Input: dimensioned drawing with shaded views. Units: mm. Origin: part minimum x, y, z. Give positions to 0.01 mm unless a question says otherwise; leave off trailing zeros. Write each loop counter-clockwise with the first axis right and the second up, starting at its lowest first coordinate (ties: lowest second). Pieces come first, ordered by that corner, then holes.
Q1. Mould query, pull axis X, two halves, no side actions, for the marked faces 1, 2 and 3. Classes: +X half, -X half, draft (parallel to the pull), parting line (faces both ways), or undercut.
Q2. Section C-C (z = 24.5). Return the cut outline in (x, y), plus the area to 3 significant figures.
Q3. Line query: line 1 (X direction, y = 50, z = 18.5); line 2 (Z direction, x = 92, y = 27). Output: solid intervals per line, ascending.
Q4. Section A-A (y = 50). Return the cut outline in (x, z).
Q5. Pin query (flat end, axial travel): pin 1 Ø10 at (x, z) = (88.5, 9.5) entering from -Y; pin 2 Ø5 at (x, z) = (76.5, 25.5) entering from +Y; pin 3 Ø2 at (y, z) = (20.5, 4) entering from -X. Return the tip coordinate at first contact, or that it passes through.
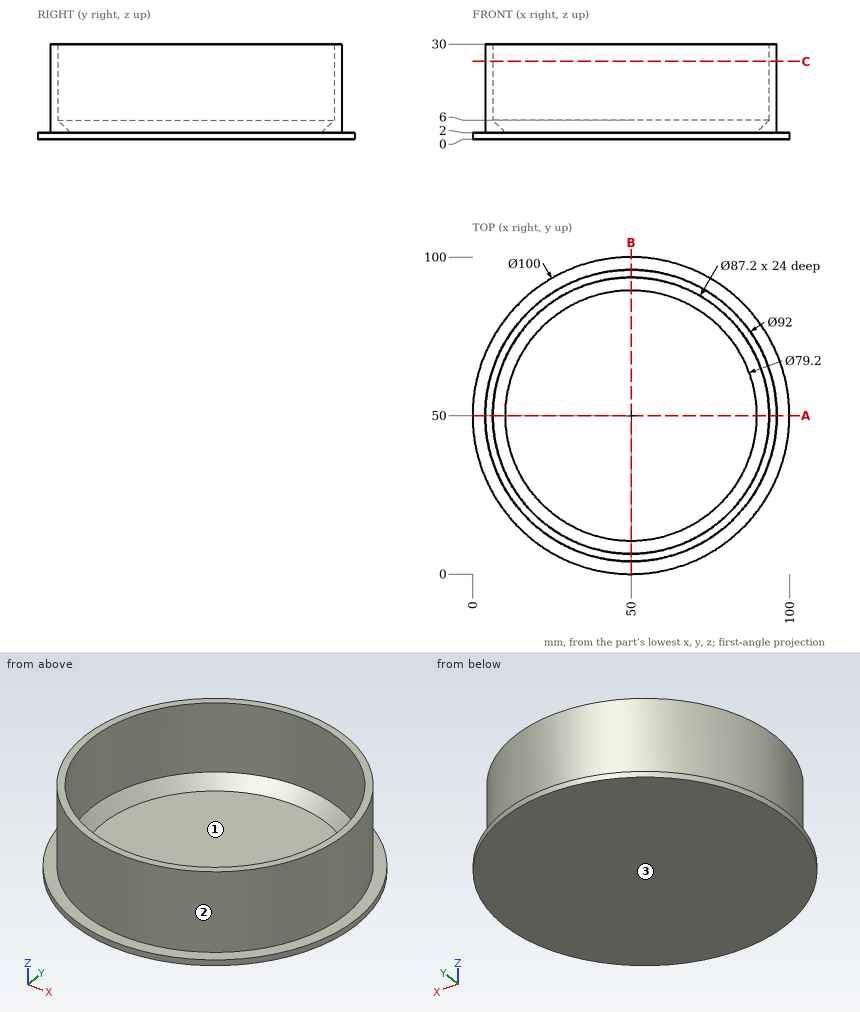
Computed:
1. face 1: undercut
1. face 2: parting line
1. face 3: draft
2. outline: circle Ø92 at (50, 50); hole circle Ø87.2 at (50, 50)
2. area: 676 mm2
3. line 1: x = 4 to 6.4, 93.6 to 96
3. line 2: z = 0 to 2
4. outline: (0, 0) - (100, 0) - (100, 2) - (96, 2) - (96, 30) - (93.6, 30) - (93.6, 6) - (89.6, 2) - (10.4, 2) - (6.4, 6) - (6.4, 30) - (4, 30) - (4, 2) - (0, 2) - close
5. pin 1: stops at y = 18.48
5. pin 2: stops at y = 89.24
5. pin 3: stops at x = 13.89
